```python
from build123d import *

# Parameters (mm, degrees)
SKETCH_W        = 28
SKETCH_H        = 26
PAD_DEPTH       = 3.5
SKETCH001_W     = 18.4
SKETCH001_H     = 21.8
POCKET_DEPTH    = 5
SKETCH002_W     = 9.4
SKETCH002_H     = 3
POCKET001_DEPTH = 5
SKETCH003_W     = 6
SKETCH003_H     = 6
POCKET002_DEPTH = 0.5
SKETCH004_R     = 0.6
POCKET003_DEPTH = 5
SKETCH010_R     = 0.8
POCKET006_DEPTH = 5
CHAMFER001_SIZE = 0.5
FILLET_R        = 1
CHAMFER002_SIZE = 1
CHAMFER003_SIZE = 0.5


with BuildPart() as part:
    # Sketch → Pad (new body, symmetric)
    with BuildSketch(Plane.XY):
        Rectangle(SKETCH_W, SKETCH_H)
    extrude(amount=PAD_DEPTH, both=True)

    # Sketch001 → Pocket (cut)
    with BuildSketch(Plane.XY.offset(-1.4)):
        Rectangle(SKETCH001_W, SKETCH001_H)
    extrude(amount=POCKET_DEPTH, mode=Mode.SUBTRACT)

    # Sketch002 → Pocket001 (cut)
    with BuildSketch(Plane.XY.offset(-0.1)):
        with Locations((0, -11.98)):
            Rectangle(SKETCH002_W, SKETCH002_H)
    extrude(amount=POCKET001_DEPTH, mode=Mode.SUBTRACT)

    # Sketch003 (on Face4 of Pocket001) → Pocket002 (cut)
    with BuildSketch(Plane(origin=(0, -7.5, -1.38), x_dir=(1, 0, 0), z_dir=(0, 0, -1))):
        Rectangle(SKETCH003_W, SKETCH003_H)
    extrude(amount=POCKET002_DEPTH, mode=Mode.SUBTRACT)

    # Sketch004 → Pocket003 (cut)
    with BuildSketch(Plane(origin=(0, -7.58, -1.3), x_dir=(1, 0, 0), z_dir=(0, 0, 1))):
        with Locations((-1.28, 1.28)):
            Circle(SKETCH004_R)
        with Locations((1.291315, 1.272746)):
            Circle(SKETCH004_R)
        with Locations((-1.28, -1.28)):
            Circle(SKETCH004_R)
        with Locations((1.28, -1.28)):
            Circle(SKETCH004_R)
    extrude(amount=-POCKET003_DEPTH, mode=Mode.SUBTRACT)

    # Sketch010 → Pocket006 (cut)
    with BuildSketch(Plane.XY.offset(-3.5)):
        with Locations((-10.923356, 0)):
            Circle(SKETCH010_R)
        with Locations((10.923356, 0)):
            Circle(SKETCH010_R)
    extrude(amount=POCKET006_DEPTH, mode=Mode.SUBTRACT)

    # Chamfer001
    chamfer001_edges = [part.edges().sort_by_distance(p)[0] for p in [
        (-9.2, 0, 3.5),
        (-4.7, -11.95, 3.5),
        (-6.95, -10.9, 3.5),
        (4.7, -11.95, 3.5),
        (6.95, -10.9, 3.5),
        (9.2, 0, 3.5),
        (0, 10.9, 3.5),
    ]]
    chamfer(chamfer001_edges, length=CHAMFER001_SIZE)

    # Fillet
    fillet_edges = [part.edges().sort_by_distance(p)[0] for p in [
        (-4.7, -11.95, -0.1),
        (4.7, -11.95, -0.1),
    ]]
    fillet(fillet_edges, radius=FILLET_R)

    # Chamfer002
    chamfer002_edges = [part.edges().sort_by_distance(p)[0] for p in [
        (14, -13, 0),
        (14, 13, 0),
        (-14, 13, 0),
        (-14, -13, 0),
    ]]
    chamfer(chamfer002_edges, length=CHAMFER002_SIZE)

    # Chamfer003
    chamfer003_edges = [part.edges().sort_by_distance(p)[0] for p in [
        (-14, 0, 3.5),
        (-13.5, -12.5, 3.5),
        (-9.1, -13, 3.5),
        (9.1, -13, 3.5),
        (13.5, -12.5, 3.5),
        (14, 0, 3.5),
        (-13.5, 12.5, 3.5),
        (0, 13, 3.5),
        (13.5, 12.5, 3.5),
    ]]
    chamfer(chamfer003_edges, length=CHAMFER003_SIZE)


solid = part.part
```
Input: part model. Units: mm. Frame: model coordinates. A direction names the side the tool comes from. Give positions to 0.01 mm unless a question says otherwise; leave off trailing zeros. Order: outer loops, then holes, each group sorted by start corner. A loop starts at its lowest first (then second) coordinate and runs counter-clockwise, first axis right, second up. Notation, with made-up numbers: (51, -29.75) - (109, -29.75) arc R24 cw to (109, -14.75) - close; hole circle Ø11 at (30, 4). An arc over 180 degrees is marked (long way). One line per item, written item: value.
1. Draft query along Y for faces 5 (the face through (-13.33, 12.32, 3.25)), 6 (the face through (13.5, -12.5, -0.3)), 7 (the face through (-9.2, 0, 1)). Return one class per face: released by +Y, released by -Y, zero draft, split by the parting line, or undercut.
Determined:
face 5: released by +Y
face 6: released by -Y
face 7: undercut
2. Cut plane C-C, the plane y = 10.25. Output: boundary loops of the cut face in (x, z).
Determined:
outline: (-14, -3.5) - (14, -3.5) - (14, 3) - (13.5, 3.5) - (9.7, 3.5) - (9.2, 3) - (9.2, -1.4) - (-9.2, -1.4) - (-9.2, 3) - (-9.7, 3.5) - (-13.5, 3.5) - (-14, 3) - close
3. Cut plane A-A, the plane y = -8.86. Output: boundary loops of the cut face in (x, z), and give its area (3 significant figures).
Determined:
outline: (-14, -3.5) - (-1.88, -3.5) - (-1.88, -1.88) - (-3, -1.88) - (-3, -1.4) - (-9.2, -1.4) - (-9.2, 3) - (-9.7, 3.5) - (-13.5, 3.5) - (-14, 3) - close; (-0.68, -3.5) - (0.68, -3.5) - (0.68, -1.88) - (-0.68, -1.88) - close; (1.88, -3.5) - (14, -3.5) - (14, 3) - (13.5, 3.5) - (9.7, 3.5) - (9.2, 3) - (9.2, -1.4) - (3, -1.4) - (3, -1.88) - (1.88, -1.88) - close
area: 98.6 mm2
4. Cut plane B-B, the plane x = -1.28. Output: boundary loops of the cut face in (y, z).
Determined:
outline: (-13, -3.5) - (-9.46, -3.5) - (-9.46, -1.88) - (-10.5, -1.88) - (-10.5, -1.4) - (-10.9, -1.4) - (-10.9, -0.1) - (-13, -0.1) - close; (-8.26, -3.5) - (-6.9, -3.5) - (-6.9, -1.88) - (-8.26, -1.88) - close; (-5.7, -3.5) - (13, -3.5) - (13, 3) - (12.5, 3.5) - (11.4, 3.5) - (10.9, 3) - (10.9, -1.4) - (-4.5, -1.4) - (-4.5, -1.88) - (-5.7, -1.88) - close
5. Pin query (flat end, axial travel): pin 1 Ø5.5 at (x, y) = (4.5, 5.5) entering from +Z; pin 2 Ø0.6 at (x, y) = (-1.5, -12) entering from +Z; pin 3 Ø1.9 at (x, y) = (1.29, -6.31) entering from +Z. Return the tip coordinate at first contact, or that it passes through.
Determined:
pin 1: z = -1.4
pin 2: z = -0.1
pin 3: z = -1.88
6. Cut plane D-D, the plane y = 0. Output: boundary loops of the cut face in (x, z).
Determined:
outline: (-14, -3.5) - (-11.72, -3.5) - (-11.72, 1.5) - (-10.12, 1.5) - (-10.12, -3.5) - (10.12, -3.5) - (10.12, 1.5) - (11.72, 1.5) - (11.72, -3.5) - (14, -3.5) - (14, 3) - (13.5, 3.5) - (9.7, 3.5) - (9.2, 3) - (9.2, -1.4) - (-9.2, -1.4) - (-9.2, 3) - (-9.7, 3.5) - (-13.5, 3.5) - (-14, 3) - close
7. Reachability of faces 1 (the face through (14, 0, 0)), 2 (the face through (11.7, 0.2, -1)), 3 (the face through (-4.7, -12, 2)), 4 (the face through (0, -8, -1.88)) from +Z, -Z, +X, -X, +Y, -Y: full face, straight path, thin tool, end or side. Return the list, or none.
Determined:
face 1: +Z, -Z, +X, +Y, -Y
face 2: -Z
face 3: +Z, -Y
face 4: +Z
8. Line query: probe 1 along Y at (x, z) = (1.28, -2.85); probe 2 along Y at (x, z) = (-11, -2); probe 3 along Y at (x, z) = (-10.5, -1). Output: solid intervals per line, ascending.
Determined:
probe 1: -13 to -9.46, -8.26 to -6.91, -5.71 to 13
probe 2: -13 to -0.8, 0.8 to 13
probe 3: -13 to -0.68, 0.68 to 13
